The drawing under review shows one solid part. Ordinate dimensions are in mm from its lowest x, y, z. Give positions to 0.01 mm unless a question says otherwise; leave off trailing zeros. Order: outer loops, then holes, each group sorted by start corner. A loop starts at its lowest first (then second) coordinate and runs counter-clockwise, first axis right, second up. Notation, with made-up numbers: M 33,11.25 L 66,11.25 A28 ccw 66,34.25 Z; hole C 23.25,73.25 d6. An arc over 180 degrees is marked long. Put each result on its own line as item: value. Start each with the question number.
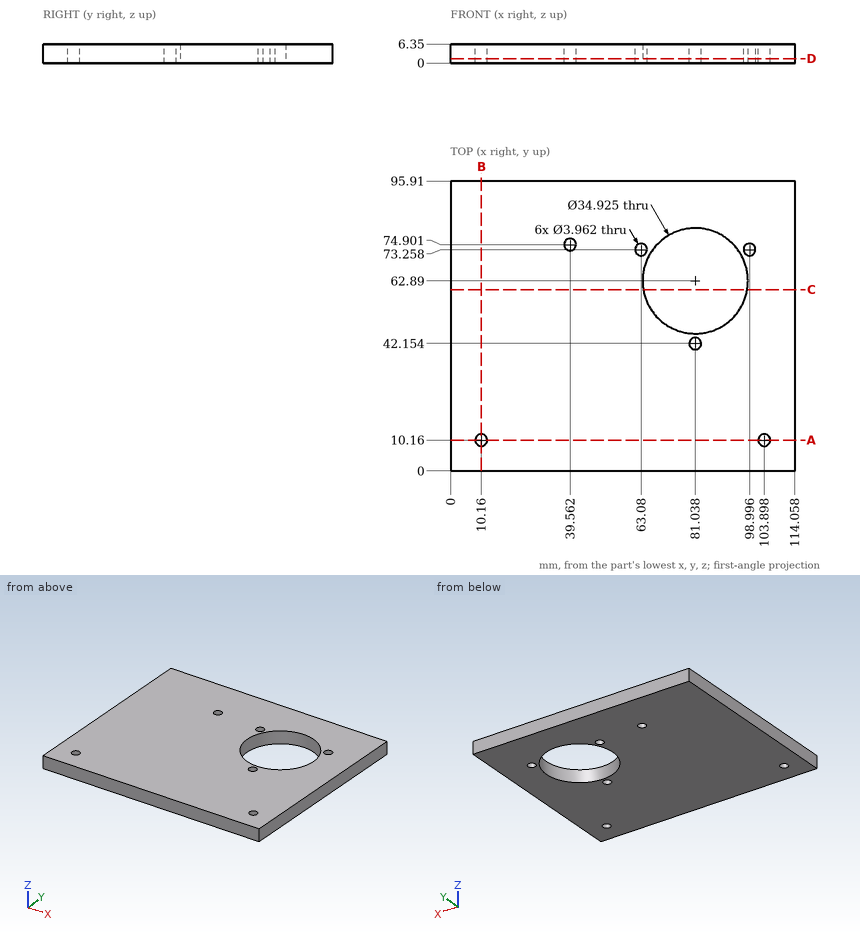
1. To check wall thickness, follow probe 1 along X at (y, z) = (10.16, 2.25); probe 2 along X at (y, z) = (63, 1.75); probe 3 along Y at (x, z) = (80, 3.75) (1 decimal). State the ranges of each line that lie inside material, in increasing order.
2. Consider section C-C on y = 60. Give the boundary of the cut face in (x, z).
3. Consider section A-A on y = 10.16. Give the boundary of the cut face in (x, z), then the cut area to 3 significant figures.
4. Consider section D-D on z = 1.5. Give the boundary of the cut face in (x, y) (1 decimal).
5. Consider section B-B on x = 10.16. Give the boundary of the cut face in (y, z), then the cut area to 3 significant figures.
Returned:
1. probe 1: x = 0 to 8.18, 12.14 to 101.92, 105.88 to 114.06
1. probe 2: x = 0 to 63.58, 98.5 to 114.06
1. probe 3: y = 0 to 40.5, 43.8 to 45.5, 80.3 to 95.9
2. outline: M 0,0 L 63.82,0 L 63.82,6.35 L 0,6.35 Z; M 98.26,0 L 114.06,0 L 114.06,6.35 L 98.26,6.35 Z
3. outline: M 0,0 L 8.18,0 L 8.18,6.35 L 0,6.35 Z; M 12.14,0 L 101.92,0 L 101.92,6.35 L 12.14,6.35 Z; M 105.88,0 L 114.06,0 L 114.06,6.35 L 105.88,6.35 Z
3. area: 674 mm2
4. outline: M 0,0 L 114.1,0 L 114.1,95.9 L 0,95.9 Z; hole C 10.2,10.2 d4; hole C 39.6,74.9 d4; hole C 63.1,73.3 d4; hole C 81,62.9 d34.9; hole C 81,42.2 d4; hole C 99,73.3 d4; hole C 103.9,10.2 d4
5. outline: M 0,0 L 8.18,0 L 8.18,6.35 L 0,6.35 Z; M 12.14,0 L 95.91,0 L 95.91,6.35 L 12.14,6.35 Z
5. area: 584 mm2
